from build123d import *

# Parameters (mm, degrees)
F0_W     = 50.8
F0_H     = 45.72
F1_DEPTH = 1.512496
F2_W     = 20.828
F2_H     = 41.148
F2_W_2   = 17.597928
F2_H_2   = 37.93566
F3_DEPTH = 19.319184


with BuildPart() as f1:
    # F0 (on Top) → F1 (new body)
    with BuildSketch(Plane.XY):
        Rectangle(F0_W, F0_H)
    extrude(amount=-F1_DEPTH)

    # F2 (on face) → F3 (join)
    with BuildSketch(Plane(origin=(0, 0, -1.512496), x_dir=(1, 0, 0), z_dir=(0, 0, -1))):
        Rectangle(F2_W, F2_H)
        Rectangle(F2_W_2, F2_H_2, mode=Mode.SUBTRACT)
    extrude(amount=F3_DEPTH)


solid = f1.part
Model file for the job. Use its own axes, mm. A direction names the side the tool comes from. Round coordinates to 2 decimals unless told otherwise and drop trailing zeros. Order: outer loops, then holes, each group sorted by start corner. A loop starts at its lowest first (then second) coordinate and runs counter-clockwise, first axis right, second up.
(1) Pull direction Y, two halves, no side cores. Call faces 6 (the face through (0, -22.86, -1)), 7 (the face through (0, 0, -1.512)), 8 (the face through (0, 20.574, -11)), 9 (the face through (-9, -2, -20.832)): released by +Y, released by -Y, zero draft, split by the parting line, or undercut.
(2) Drill centre lines: line 1 (X direction, y = 0.5, z = -18.75); line 2 (Y direction, x = -1.5, z = -17); line 3 (Z direction, x = -7, y = 4). Where is each one in solid material? Low to high.
(3) Band-saw the part on A-A (z = -14.75). List the corners of the cut face in (x, y).
(4) Band-saw the part on D-D (x = 16.5). List the corners of the cut face in (y, z).
(5) 3-axis set-ups, long thin cutter, end or side, ignore diameter. For faces 1 (the face through (10.414, 0, -11)), 2 (the face through (0, -20.574, -11)), 3 (the face through (-8.799, 0, -11)), 4 (the face through (0, 22.86, -1)), 5 (the face through (-10.414, 0, -11)): which of +Z, -Z, +X, -X, +Y, -Y reach the whole face in a straight line?
(6) Pin check, flat tips, straight feed: pin 1 (6 mm diameter, centred on x = -1.5, z = -10, fed in from -Y); pin 2 (6 mm diameter, centred on y = 6, z = -10.5, fed in from +X); pin 3 (5 mm diameter, centred on x = 13, z = -16, fed in from +Y); pin 4 (4 mm diameter, centred on x = -5, y = -16, fed in from -Z). Stop position of each tip, or through.
(7) Band-saw the part on C-C (y = 15). List the corners of the cut face in (x, z).
(8) Band-saw the part on B-B (x = 5.5). List the corners of the cut face in (y, z), then the cut area to 3 significant figures.
Verdict:
1. face 6: released by -Y
1. face 7: undercut
1. face 8: released by +Y
1. face 9: zero draft
2. line 1: x = -10.41 to -8.8, 8.8 to 10.41
2. line 2: y = -20.57 to -18.97, 18.97 to 20.57
2. line 3: z = -1.51 to 0
3. outline: (-10.41, -20.57) - (10.41, -20.57) - (10.41, 20.57) - (-10.41, 20.57) - close; hole (-8.8, -18.97) - (8.8, -18.97) - (8.8, 18.97) - (-8.8, 18.97) - close
4. outline: (-22.86, -1.51) - (22.86, -1.51) - (22.86, 0) - (-22.86, 0) - close
5. face 1: -Z, +X, +Y, -Y
5. face 2: -Z, +X, -X, -Y
5. face 3: -Z
5. face 4: +Z, -Z, +X, -X, +Y
5. face 5: -Z, -X, +Y, -Y
6. pin 1: stops at y = -20.57
6. pin 2: stops at x = 10.41
6. pin 3: passes through
6. pin 4: stops at z = -1.51
7. outline: (-25.4, -1.51) - (-10.41, -1.51) - (-10.41, -20.83) - (-8.8, -20.83) - (-8.8, -1.51) - (8.8, -1.51) - (8.8, -20.83) - (10.41, -20.83) - (10.41, -1.51) - (25.4, -1.51) - (25.4, 0) - (-25.4, 0) - close
8. outline: (-22.86, -1.51) - (-20.57, -1.51) - (-20.57, -20.83) - (-18.97, -20.83) - (-18.97, -1.51) - (18.97, -1.51) - (18.97, -20.83) - (20.57, -20.83) - (20.57, -1.51) - (22.86, -1.51) - (22.86, 0) - (-22.86, 0) - close
8. area: 131 mm2
